Design review of the part shown in the three views and the two pictorial views. Dimensions are in mm from the part's minimum x, y and z. Give positions to 0.01 mm unless a question says otherwise; leave off trailing zeros. Write each loop counter-clockwise with the first axis right and the second up, starting at its lowest first coordinate (ties: lowest second). Pieces come first, ordered by that corner, then holes. Notation, with made-up numbers: (87.5, 10) -> (140.5, 10) arc R22 ccw to (140.5, 26) -> close; hole circle Ø11 at (60, 23.5). An arc over 180 degrees is marked (long way). Return JSON: item names as keys, results as strings. Group by question number.
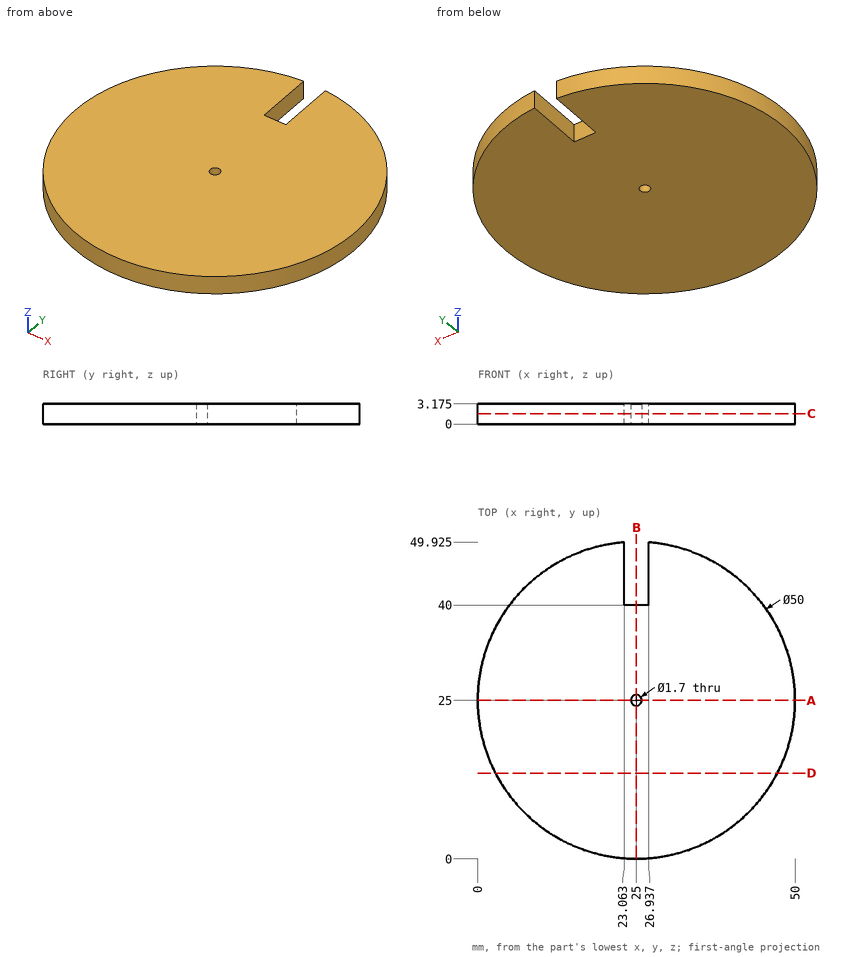
Q1. Insertion check: pin 1 (1 mm diameter, centred on x = 20, z = 3, fed in from -Y); pin 2 (1 mm diameter, centred on y = 43.5, z = 2, fed in from -X); pin 3 (1.5 mm diameter, centred on x = 26, z = 0.5, fed in from +Y). Each pin has a flat end and moves straight along its axis. Give the tip position at first contact, or say it passes through.
Q2. Take a section at D-D, the plane y = 13.5. Give the boundary of the cut face in (x, z) (3 decimals).
Q3. Take a section at A-A, the plane y = 25. Give the boundary of the cut face in (x, z) (3 decimals), plus the area to 3 significant figures.
Q4. For L1, parallel to Y at x = 25, z = 2.4; L2, parallel to Y at x = 26.5, z = 0.15 (3 decimals); L3, parallel to Y at x = 36, z = 2.65, list the stretches that pass through material, from the lowest coordinate up. Write a range as from..to.
Q5. Take a section at B-B, the plane x = 25. Give the boundary of the cut face in (y, z) (3 decimals).
Q6. Take a section at C-C, the plane z = 1.65. Give the boundary of the cut face in (x, y) (3 decimals), plus the area to 3 significant figures.
Final values:
{
 "1": {"pin 1": "stops at y = 0.41", "pin 2": "stops at x = 7.65", "pin 3": "stops at y = 40"},
 "2": {"outline": "(2.802, 0) -> (47.198, 0) -> (47.198, 3.175) -> (2.802, 3.175) -> close"},
 "3": {"outline": "(0, 0) -> (24.15, 0) -> (24.15, 3.175) -> (0, 3.175) -> close; (25.85, 0) -> (50, 0) -> (50, 3.175) -> (25.85, 3.175) -> close", "area": "153 mm²"},
 "4": {"L1": "y = 0..24.15, 25.85..40", "L2": "y = 0.045..40", "L3": "y = 2.55..47.45"},
 "5": {"outline": "(0, 0) -> (24.15, 0) -> (24.15, 3.175) -> (0, 3.175) -> close; (25.85, 0) -> (40, 0) -> (40, 3.175) -> (25.85, 3.175) -> close"},
 "6": {"outline": "(23.063, 40) -> (23.063, 49.925) arc R25 ccw (long way) to (26.937, 49.925) -> (26.937, 40) -> close; hole circle Ø1.7 at (25, 25)", "area": "1,920 mm²"}
}
